```python
from build123d import *

# Parameters (mm, degrees)
SKETCH_1_W             = 38
SKETCH_1_H             = 21
EXTRUDE_1_DEPTH        = 3
SKETCH_2_R             = 1.3
CUT_EXTRUDE_1_DEPTH    = 3
PATTERN_LINEAR_1_COUNT = 2
PATTERN_LINEAR_1_PITCH = 24
SKETCH_9_W             = 15
SKETCH_9_H             = 21
EXTRUDE_5_DEPTH        = 40
SKETCH_10_R            = 5
CUT_EXTRUDE_5_DEPTH    = 60
SKETCH_11_W            = 6
SKETCH_11_H            = 21
CUT_EXTRUDE_6_DEPTH    = 35
SKETCH_12_R            = 6
EXTRUDE_6_DEPTH        = 2
SKETCH_14_R            = 6
EXTRUDE_8_DEPTH        = 2
SKETCH_15_R            = 2.5
CUT_EXTRUDE_7_DEPTH    = 20
SKETCH_16_W            = 15
SKETCH_16_H            = 50.5
EXTRUDE_9_DEPTH        = 5
FILLET_START           = -41.833744856
FILLET_2_DEPTH         = 38
FILLET_START_2         = -30.333744856
FILLET_2_2_DEPTH       = 4.5
FILLET_START_3         = -19.833744856
FILLET_2_3_DEPTH       = 4.5
FILLET_3_R             = 5
SKETCH_17_W            = 6
SKETCH_17_H            = 22
CUT_EXTRUDE_8_DEPTH    = 100


with BuildPart() as part:
    # 草图1 → 凸台-拉伸1 (new body)
    with BuildSketch(Plane.XY):
        with Locations((-22.833744856, 0.637037037)):
            Rectangle(SKETCH_1_W, SKETCH_1_H)
    extrude(amount=EXTRUDE_1_DEPTH)

    # 草图2 → 切除-拉伸1 (cut)
    with BuildSketch(Plane(origin=(0, 0, 0), x_dir=(-1, 0, 0), z_dir=(0, 0, -1))):
        with Locations((10.833744856, 6.637037037)):
            Circle(SKETCH_2_R)
        with Locations((10.833744856, -5.362962963)):
            Circle(SKETCH_2_R)
    cut_extrude_1 = extrude(amount=-CUT_EXTRUDE_1_DEPTH, mode=Mode.SUBTRACT)

    # 阵列(线性)1: 切除-拉伸1 ×2
    with Locations(*[(-i * PATTERN_LINEAR_1_PITCH, 0, 0) for i in range(1, PATTERN_LINEAR_1_COUNT)]):
        add(cut_extrude_1, mode=Mode.SUBTRACT)

    # 草图9 → 凸台-拉伸5 (add)
    with BuildSketch(Plane(origin=(0, 0, 0), x_dir=(-1, 0, 0), z_dir=(0, 0, -1))):
        with Locations((22.833744856, 0.637037037)):
            Rectangle(SKETCH_9_W, SKETCH_9_H)
    extrude(amount=EXTRUDE_5_DEPTH)

    # 草图10 → 切除-拉伸5 (cut)
    with BuildSketch(Plane(origin=(-15.333744856, 0, 0), x_dir=(0, 0, -1), z_dir=(1, 0, 0))):
        with Locations(Location((30, 0.637037037, 0), (0, 0, 90))):
            Circle(SKETCH_10_R)
    extrude(amount=-CUT_EXTRUDE_5_DEPTH, mode=Mode.SUBTRACT)

    # 草图11 → 切除-拉伸6 (cut)
    with BuildSketch(Plane(origin=(0, 0, -40), x_dir=(-1, 0, 0), z_dir=(0, 0, -1))):
        with Locations((22.833744856, 0.637037037)):
            Rectangle(SKETCH_11_W, SKETCH_11_H)
    extrude(amount=-CUT_EXTRUDE_6_DEPTH, mode=Mode.SUBTRACT)

    # 草图12 → 凸台-拉伸6 (add)
    with BuildSketch(Plane.ZY.offset(19.833744856)):
        with Locations((-30, 0.637037037)):
            Circle(SKETCH_12_R)
    extrude(amount=-EXTRUDE_6_DEPTH)

    # 草图14 → 凸台-拉伸8 (add)
    with BuildSketch(Plane(origin=(-25.833744856, 0, 0), x_dir=(0, 0, -1), z_dir=(1, 0, 0))):
        with Locations((30, 0.637037037)):
            Circle(SKETCH_14_R)
    extrude(amount=-EXTRUDE_8_DEPTH)

    # 草图15 → 切除-拉伸7 (cut)
    with BuildSketch(Plane(origin=(-17.833744856, 0, 0), x_dir=(0, 0, -1), z_dir=(1, 0, 0))):
        with Locations(Location((30, 0.637037037, 0), (0, 0, 90))):
            Circle(SKETCH_15_R)
    extrude(amount=-CUT_EXTRUDE_7_DEPTH, mode=Mode.SUBTRACT)

    # 草图16 → 凸台-拉伸9 (add)
    with BuildSketch(Plane(origin=(0, -9.862962963, 0), x_dir=(-1, 0, 0), z_dir=(0, -1, 0))):
        with Locations((22.833744856, 25.25)):
            Rectangle(SKETCH_16_W, SKETCH_16_H)
    extrude(amount=EXTRUDE_9_DEPTH)

    # 圆角2: read off the stored shape, not the designer's step
    # 圆角2 outline → 圆角2 (cut)
    with BuildSketch(Plane.YZ.offset(FILLET_START)):
        with BuildLine():
            Line((11.137037037, -40), (11.137037037, -29.5))
            ThreePointArc((11.137037037, -29.5), (8.061658239, -36.924621202), (0.637037037, -40))
            Line((0.637037037, -40), (11.137037037, -40))
        make_face()
    extrude(amount=FILLET_2_DEPTH, mode=Mode.SUBTRACT)

    # Fillet 2 2 outline → Fillet 2 2 (add)
    with BuildSketch(Plane.YZ.offset(FILLET_START_2)):
        with BuildLine():
            ThreePointArc((-9.862962963, -50.5), (-6.787584165, -43.075378798), (0.637037037, -40))
            Line((0.637037037, -40), (-9.862962963, -40))
            Line((-9.862962963, -40), (-9.862962963, -50.5))
        make_face()
    extrude(amount=FILLET_2_2_DEPTH)

    # Fillet 2 3 outline → Fillet 2 3 (add)
    with BuildSketch(Plane.YZ.offset(FILLET_START_3)):
        with BuildLine():
            ThreePointArc((-9.862962963, -50.5), (-6.787584165, -43.075378798), (0.637037037, -40))
            Line((0.637037037, -40), (-9.862962963, -40))
            Line((-9.862962963, -40), (-9.862962963, -50.5))
        make_face()
    extrude(amount=FILLET_2_3_DEPTH)

    # 圆角3
    fillet_3_edges = [part.edges().sort_by_distance(p)[0] for p in [
        (-22.833744856, -14.862962963, 0),
    ]]
    fillet(fillet_3_edges, radius=FILLET_3_R - 0.0001)  # a hair under: the kernel refuses the full size

    # 草图17 → 切除-拉伸8 (cut)
    with BuildSketch(Plane(origin=(0, 0, -5), x_dir=(-1, 0, 0), z_dir=(0, 0, -1))):
        with Locations((22.833744856, 0.137037037)):
            Rectangle(SKETCH_17_W, SKETCH_17_H)
    extrude(amount=CUT_EXTRUDE_8_DEPTH, mode=Mode.SUBTRACT)


solid = part.part
```
Input: part model. Units: mm. Frame: model coordinates. A direction names the side the tool comes from. Give positions to 0.01 mm unless a question says otherwise; leave off trailing zeros. Order: outer loops, then holes, each group sorted by start corner. A loop starts at its lowest first (then second) coordinate and runs counter-clockwise, first axis right, second up. Notation, with made-up numbers: (-32.75, 88) - (-6.75, 88) arc R19 ccw to (-6.75, 125) - close; hole circle Ø7 at (18.5, 34). An arc over 180 degrees is marked (long way). Put each result on its own line as item: value.
Item 1: Access query for faces 5 (the flat face through (-17.834, -2, -28)), 6 (the flat face through (-30.334, -2, -19)), 7 (the flat face through (-15.334, -2, -19)). Directions: +Z, -Z, +X, -X, +Y, -Y. A direction counts if a zero-diameter tool reaches every point of the face in a straight line with its end or side. Return the directions, or none.
Found:
face 5: +X
face 6: -Z, -X, +Y, -Y
face 7: -Z, +X, +Y, -Y
Item 2: Draft query along X for faces 1 (the cylindrical face through (-18.82, 0.31, -27.52)), 2 (the flat face through (-27.834, -2, -32)), 3 (the cylindrical face through (-35.533, 7.733, 1.479)), 4 (the cylindrical face through (-35.533, -4.267, 1.479)). Return one class per face: +X half, -X half, draft (parallel to the pull), parting line (faces both ways), or undercut.
Found:
face 1: draft
face 2: -X half
face 3: undercut
face 4: undercut
Item 3: Contact query for flat-ended pins moving along their axis: pin 1 (3 mm diameter, centred on y = -1.5, z = -29, fed in from +X); pin 2 (2 mm diameter, centred on y = -11, z = -25.5, fed in from +X); pin 3 (13 mm diameter, centred on y = -1.5, z = -20, fed in from -X); pin 4 (2 mm diameter, centred on x = -34.83, y = 6.64, fed in from +Z). Output: stop coordinate, or through.
Found:
pin 1: stops at x = -17.83
pin 2: stops at x = -15.33
pin 3: stops at x = -30.33
pin 4: passes through
Item 4: Section query D-D, the plane x = -39. Return loops of the section in (y, z).
Found:
outline: (-9.86, 0) - (11.14, 0) - (11.14, 3) - (-9.86, 3) - close
Item 5: Ray query, L1, parallel to X at y = 1.25, z = -7; L2, parallel to Z at x = -31.5, y = -0.5; L3, parallel to Y at x = -24, z = -18. Return the intervals inside material, ascending. Write a range as from..to.
Found:
L1: x = -30.33..-25.83, -19.83..-15.33
L2: z = 0..3
L3: y = -14.86..-10.86
Item 6: Section query B-B, the plane z = -20.5. Return loops of the section in (x, y), then the cut area to 3 significant figures.
Found:
outline: (-30.33, -14.86) - (-15.33, -14.86) - (-15.33, 11.14) - (-19.83, 11.14) - (-19.83, -10.86) - (-25.83, -10.86) - (-25.83, 11.14) - (-30.33, 11.14) - close
area: 258 mm^2
